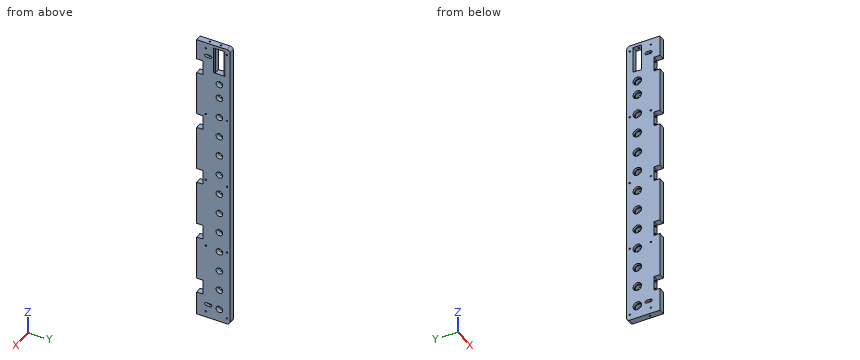
```python
from build123d import *

# Parameters (mm, degrees)
SKETCH1_W                 = 1000
SKETCH1_H                 = 100
SKETCH1_R                 = 11
SKETCH1_W_2               = 90
SKETCH1_H_2               = 28
BOSS_EXTRUDE1_DEPTH       = 20
SKETCH2_W                 = 20
SKETCH2_H                 = 50
SKETCH2_R                 = 4
CUT_EXTRUDE2_DEPTH        = 20
LPATTERN1_COUNT           = 2
LPATTERN1_PITCH           = 220
SKETCH12_R                = 14
CUT_EXTRUDE6_DEPTH        = 8
SKETCH14_W                = 2.5
SKETCH14_H                = 10
SKETCH16_W                = 90
SKETCH16_H                = 5
CUT_EXTRUDE7_DEPTH        = 3
SKETCH17_W                = 90
SKETCH17_H                = 5
CUT_EXTRUDE8_DEPTH        = 3
SKETCH18_R                = 14
CUT_EXTRUDE9_DEPTH        = 8
SKETCH20_W                = 20
SKETCH20_H                = 1000
BOSS_EXTRUDE2_DEPTH       = 10
FILLET1_R                 = 10
FILLET2_R                 = 10
F_5_0MM_DOWEL_HOLE3_D     = 5
F_5_0MM_DOWEL_HOLE3_DEPTH = 10
F_5_0MM_DOWEL_HOLE3_TIP   = 1.502151548
SKETCH27_R                = 2.5
CUT_EXTRUDE10_DEPTH       = 55
CUT_EXTRUDE11_DEPTH       = 1035.26302264
CUT_EXTRUDE12_START       = -70
SKETCH29_R                = 2.5
CUT_EXTRUDE12_DEPTH       = 70
SKETCH30_R                = 2.5
CUT_EXTRUDE13_DEPTH       = 1035.26302264
CUT_EXTRUDE14_REACH       = 1036.263
SKETCH31_W                = 1251.907534991
SKETCH31_H                = 393.114099754
SKETCH32_R                = 4
CUT_EXTRUDE15_DEPTH       = 35


with BuildPart() as part:
    # Sketch1 → Boss-Extrude1 (new body)
    with BuildSketch(Plane(origin=(0, 0, 0), x_dir=(0, 0, -1), z_dir=(1, 0, 0))):
        with Locations((500, 50)):
            Rectangle(SKETCH1_W, SKETCH1_H)
        with Locations((956.5, 75)):
            Circle(SKETCH1_R, mode=Mode.SUBTRACT)
        with Locations((886.5, 75)):
            Circle(SKETCH1_R, mode=Mode.SUBTRACT)
        with Locations((816.5, 75)):
            Circle(SKETCH1_R, mode=Mode.SUBTRACT)
        with Locations((746.5, 75)):
            Circle(SKETCH1_R, mode=Mode.SUBTRACT)
        with Locations((676.5, 75)):
            Circle(SKETCH1_R, mode=Mode.SUBTRACT)
        with Locations((606.5, 75)):
            Circle(SKETCH1_R, mode=Mode.SUBTRACT)
        with Locations((536.5, 75)):
            Circle(SKETCH1_R, mode=Mode.SUBTRACT)
        with Locations((466.5, 75)):
            Circle(SKETCH1_R, mode=Mode.SUBTRACT)
        with Locations((396.5, 75)):
            Circle(SKETCH1_R, mode=Mode.SUBTRACT)
        with Locations((326.5, 75)):
            Circle(SKETCH1_R, mode=Mode.SUBTRACT)
        with Locations((256.5, 75)):
            Circle(SKETCH1_R, mode=Mode.SUBTRACT)
        with Locations((186.5, 75)):
            Circle(SKETCH1_R, mode=Mode.SUBTRACT)
        with Locations((136.5, 75)):
            Circle(SKETCH1_R, mode=Mode.SUBTRACT)
        with Locations((55, 75)):
            Rectangle(SKETCH1_W_2, SKETCH1_H_2, mode=Mode.SUBTRACT)
    extrude(amount=BOSS_EXTRUDE1_DEPTH)

    # Sketch2 → Cut-Extrude2 (cut)
    # profile 1 of 5: a face of its own
    with BuildSketch(Plane.XZ):
        with Locations((10, -895)):
            Rectangle(SKETCH2_W, SKETCH2_H)
        with Locations(Location((10, -910, 0), (0, 0, 270))):
            Circle(SKETCH2_R, mode=Mode.SUBTRACT)
        with Locations(Location((10, -880, 0), (0, 0, 270))):
            Circle(SKETCH2_R, mode=Mode.SUBTRACT)
    # profile 2 of 5: a face of its own
    with BuildSketch(Plane.XZ):
        with Locations((10, -695)):
            Rectangle(SKETCH2_W, SKETCH2_H)
        with Locations(Location((10, -710, 0), (0, 0, 270))):
            Circle(SKETCH2_R, mode=Mode.SUBTRACT)
        with Locations(Location((10, -680, 0), (0, 0, 270))):
            Circle(SKETCH2_R, mode=Mode.SUBTRACT)
    # profile 3 of 5: a face of its own
    with BuildSketch(Plane.XZ):
        with Locations((10, -495)):
            Rectangle(SKETCH2_W, SKETCH2_H)
        with Locations(Location((10, -510, 0), (0, 0, 270))):
            Circle(SKETCH2_R, mode=Mode.SUBTRACT)
        with Locations(Location((10, -480, 0), (0, 0, 270))):
            Circle(SKETCH2_R, mode=Mode.SUBTRACT)
    # profile 4 of 5: a face of its own
    with BuildSketch(Plane.XZ):
        with Locations((10, -295)):
            Rectangle(SKETCH2_W, SKETCH2_H)
        with Locations(Location((10, -310, 0), (0, 0, 270))):
            Circle(SKETCH2_R, mode=Mode.SUBTRACT)
        with Locations(Location((10, -280, 0), (0, 0, 270))):
            Circle(SKETCH2_R, mode=Mode.SUBTRACT)
    # profile 5 of 5: a face of its own
    with BuildSketch(Plane.XZ):
        with Locations((10, -95)):
            Rectangle(SKETCH2_W, SKETCH2_H)
        with Locations(Location((10, -110, 0), (0, 0, 270))):
            Circle(SKETCH2_R, mode=Mode.SUBTRACT)
        with Locations(Location((10, -80, 0), (0, 0, 270))):
            Circle(SKETCH2_R, mode=Mode.SUBTRACT)
    extrude(amount=-CUT_EXTRUDE2_DEPTH, mode=Mode.SUBTRACT)


with BuildPart() as lpattern1_1:
    # LPattern1: pattern copy
    add(part.part.moved(Location(Vector(-1, 0, 0) * (1 * LPATTERN1_PITCH))))

    # Sketch12 → Cut-Extrude6 (cut)
    with BuildSketch(Plane(origin=(-200, 0, 0), x_dir=(0, 0, -1), z_dir=(1, 0, 0))):
        with Locations((956.5, 75)):
            Circle(SKETCH12_R)
        with Locations((886.5, 75)):
            Circle(SKETCH12_R)
        with Locations((816.5, 75)):
            Circle(SKETCH12_R)
        with Locations((746.5, 75)):
            Circle(SKETCH12_R)
        with Locations((676.5, 75)):
            Circle(SKETCH12_R)
        with Locations((606.5, 75)):
            Circle(SKETCH12_R)
        with Locations((536.5, 75)):
            Circle(SKETCH12_R)
        with Locations((466.5, 75)):
            Circle(SKETCH12_R)
        with Locations((396.5, 75)):
            Circle(SKETCH12_R)
        with Locations((326.5, 75)):
            Circle(SKETCH12_R)
        with Locations((256.5, 75)):
            Circle(SKETCH12_R)
        with Locations((186.5, 75)):
            Circle(SKETCH12_R)
        with Locations((136.5, 75)):
            Circle(SKETCH12_R)
    extrude(amount=-CUT_EXTRUDE6_DEPTH, mode=Mode.SUBTRACT)

    # Sketch16 → Cut-Extrude7 (cut)
    with BuildSketch(Plane.ZY.offset(220)):
        with Locations((-55, 91.5)):
            Rectangle(SKETCH16_W, SKETCH16_H)
        with Locations((-55, 58.5)):
            Rectangle(SKETCH16_W, SKETCH16_H)
    extrude(amount=-CUT_EXTRUDE7_DEPTH, mode=Mode.SUBTRACT)


with BuildPart() as part_1:
    add(part.part)

    # Sketch14 → Ø5.0mm Dowel Hole1 (revolve, cut)
    with BuildSketch(Plane(origin=(10, 75, 0), x_dir=(0, -1, 0), z_dir=(1, 0, 0))):
        with Locations((1.25, 5)):
            Rectangle(SKETCH14_W, SKETCH14_H)
    revolve(axis=Axis((10, 75, 6.35), (0, 0, -1)), mode=Mode.SUBTRACT)

    # Sketch17 → Cut-Extrude8 (cut)
    with BuildSketch(Plane(origin=(20, 0, 0), x_dir=(0, 0, -1), z_dir=(1, 0, 0))):
        with Locations((55, 91.5)):
            Rectangle(SKETCH17_W, SKETCH17_H)
        with Locations((55, 58.5)):
            Rectangle(SKETCH17_W, SKETCH17_H)
    extrude(amount=-CUT_EXTRUDE8_DEPTH, mode=Mode.SUBTRACT)

    # Sketch18 → Cut-Extrude9 (cut)
    with BuildSketch(Plane.ZY):
        with Locations((-956.5, 75)):
            Circle(SKETCH18_R)
        with Locations((-886.5, 75)):
            Circle(SKETCH18_R)
        with Locations((-816.5, 75)):
            Circle(SKETCH18_R)
        with Locations((-746.5, 75)):
            Circle(SKETCH18_R)
        with Locations((-676.5, 75)):
            Circle(SKETCH18_R)
        with Locations((-606.5, 75)):
            Circle(SKETCH18_R)
        with Locations((-536.5, 75)):
            Circle(SKETCH18_R)
        with Locations((-466.5, 75)):
            Circle(SKETCH18_R)
        with Locations((-396.5, 75)):
            Circle(SKETCH18_R)
        with Locations((-326.5, 75)):
            Circle(SKETCH18_R)
        with Locations((-256.5, 75)):
            Circle(SKETCH18_R)
        with Locations((-186.5, 75)):
            Circle(SKETCH18_R)
        with Locations((-136.5, 75)):
            Circle(SKETCH18_R)
    extrude(amount=-CUT_EXTRUDE9_DEPTH, mode=Mode.SUBTRACT)

    add(lpattern1_1.part)  # Boss-Extrude2 merges LPattern1_1
    # Sketch20 → Boss-Extrude2 (add)
    with BuildSketch(Plane(origin=(0, 100, 0), x_dir=(1, 0, 0), z_dir=(0, 1, 0))):
        with Locations((-210, 500)):
            Rectangle(SKETCH20_W, SKETCH20_H)
        with Locations((10, 500)):
            Rectangle(SKETCH20_W, SKETCH20_H)
    extrude(amount=BOSS_EXTRUDE2_DEPTH)

    # Fillet1
    fillet1_edges = [part_1.edges().sort_by_distance(p)[0] for p in [
        (-210, 110, 0),
        (-210, 110, -1000),
    ]]
    fillet(fillet1_edges, radius=FILLET1_R)

    # Fillet2
    fillet2_edges = [part_1.edges().sort_by_distance(p)[0] for p in [
        (10, 110, 0),
        (10, 110, -1000),
    ]]
    fillet(fillet2_edges, radius=FILLET2_R)

    # Ø5.0mm Dowel Hole3
    with Locations(Plane(origin=(-210, 74.987891575, 0), x_dir=(1, 0, 0), z_dir=(0, 0, 1))):
        with Locations((0, 0)):
            Hole(F_5_0MM_DOWEL_HOLE3_D / 2, depth=F_5_0MM_DOWEL_HOLE3_DEPTH)
            with Locations((0, 0, -(F_5_0MM_DOWEL_HOLE3_DEPTH + F_5_0MM_DOWEL_HOLE3_TIP / 2))):  # 118° drill point
                Cone(0, F_5_0MM_DOWEL_HOLE3_D / 2, F_5_0MM_DOWEL_HOLE3_TIP, mode=Mode.SUBTRACT)

    # Sketch27 → Cut-Extrude10 (cut)
    with BuildSketch(Plane.XY):
        with Locations((-210, 38)):
            Circle(SKETCH27_R)
        with Locations((10, 38)):
            Circle(SKETCH27_R)
    extrude(amount=-CUT_EXTRUDE10_DEPTH, mode=Mode.SUBTRACT)

    # Sketch28 → Cut-Extrude11 (cut, through all)
    with BuildSketch(Plane.ZY.offset(220)):
        with BuildLine():
            Line((-42, 44.831263619), (-42, 31.168736381))
            ThreePointArc((-42, 31.168736381), (-47, 26.168736381), (-52, 31.168736381))
            Line((-52, 31.168736381), (-52, 44.831263619))
            ThreePointArc((-52, 44.831263619), (-47, 49.831263619), (-42, 44.831263619))
        make_face()
        with BuildLine():
            Line((-958, 44.831263619), (-958, 31.168736381))
            ThreePointArc((-958, 31.168736381), (-953, 26.168736381), (-948, 31.168736381))
            Line((-948, 31.168736381), (-948, 44.831263619))
            ThreePointArc((-948, 44.831263619), (-953, 49.831263619), (-958, 44.831263619))
        make_face()
    extrude(amount=-CUT_EXTRUDE11_DEPTH, mode=Mode.SUBTRACT)

    # Sketch29 → Cut-Extrude12 (cut)
    with BuildSketch(Plane(origin=(0, 0, -1000), x_dir=(-1, 0, 0), z_dir=(0, 0, -1)).offset(CUT_EXTRUDE12_START)):
        with Locations(Location((-10, 38, 0), (0, 0, 180))):
            Circle(SKETCH29_R)
        with Locations(Location((210, 38, 0), (0, 0, 180))):
            Circle(SKETCH29_R)
    extrude(amount=CUT_EXTRUDE12_DEPTH, mode=Mode.SUBTRACT)

    # Sketch30 → Cut-Extrude13 (cut, through all)
    with BuildSketch(Plane(origin=(20, 0, 0), x_dir=(0, 0, -1), z_dir=(1, 0, 0))):
        with Locations((500, 30)):
            Circle(SKETCH30_R)
        with Locations((20, 30)):
            Circle(SKETCH30_R)
        with Locations((20, 100)):
            Circle(SKETCH30_R)
        with Locations((500, 100)):
            Circle(SKETCH30_R)
        with Locations((980, 100)):
            Circle(SKETCH30_R)
        with Locations((980, 30)):
            Circle(SKETCH30_R)
        with Locations((260, 100)):
            Circle(SKETCH30_R)
        with Locations((740, 100)):
            Circle(SKETCH30_R)
        with Locations((740, 30)):
            Circle(SKETCH30_R)
        with Locations((260, 30)):
            Circle(SKETCH30_R)
    extrude(amount=-CUT_EXTRUDE13_DEPTH, mode=Mode.SUBTRACT)

    # Sketch31 → Cut-Extrude14 (cut, up to next)
    with BuildSketch(Plane.ZY.offset(220), mode=Mode.PRIVATE) as cut_extrude14_sk1:
        with Locations((-530.819455446, 0)):
            Rectangle(SKETCH31_W, SKETCH31_H)
    cut_extrude14_tool1 = extrude(cut_extrude14_sk1.sketch, amount=-CUT_EXTRUDE14_REACH, mode=Mode.PRIVATE) & part_1.part
    add(cut_extrude14_tool1.solids().sort_by_distance((-220, 0, -530.819455))[0], mode=Mode.SUBTRACT)

    # Sketch32 → Cut-Extrude15 (cut)
    with BuildSketch(Plane.XZ):
        with Locations(Location((10, -310, 0), (0, 0, 270))):
            Circle(SKETCH32_R)
        with Locations(Location((10, -280, 0), (0, 0, 270))):
            Circle(SKETCH32_R)
        with Locations(Location((10, -110, 0), (0, 0, 270))):
            Circle(SKETCH32_R)
        with Locations(Location((10, -80, 0), (0, 0, 270))):
            Circle(SKETCH32_R)
        with Locations(Location((10, -480, 0), (0, 0, 270))):
            Circle(SKETCH32_R)
        with Locations(Location((10, -510, 0), (0, 0, 270))):
            Circle(SKETCH32_R)
        with Locations(Location((10, -680, 0), (0, 0, 270))):
            Circle(SKETCH32_R)
        with Locations(Location((10, -710, 0), (0, 0, 270))):
            Circle(SKETCH32_R)
        with Locations(Location((10, -880, 0), (0, 0, 270))):
            Circle(SKETCH32_R)
        with Locations(Location((10, -910, 0), (0, 0, 270))):
            Circle(SKETCH32_R)
    extrude(amount=-CUT_EXTRUDE15_DEPTH, mode=Mode.SUBTRACT)


solid = part_1.part
```
Work out the finished part from the listing and answer in its coordinate system (mm). Coordinates: 2 decimals unless noted, no trailing zeros. Order: outer loops, then holes, each group sorted by start corner. A loop starts at its lowest first (then second) coordinate and runs counter-clockwise, first axis right, second up. Notation, with made-up numbers: (-21, 2) - (22, 2) arc R22 cw to (22, 30) - close; hole circle Ø7 at (71, -2.5). An arc over 180 degrees is marked (long way). Answer as a JSON object with one key per item and string values.
1. Find section A-A on z = -136.5. Determine the outline of the cut face in (x, y).
Output values:
{"outline": "(0, 0) - (20, 0) - (20, 64) - (8, 64) - (8, 61) - (0, 61) - close; (0, 89) - (8, 89) - (8, 86) - (20, 86) - (20, 110) - (0, 110) - close"}
2. Each of these flat-tipped pins is pushed along its axis until it touches: P1, Ø1.5, axis at x = 10.5, y = 38.5, coming from the -Z side; P2, Ø10.5, axis at x = 10, z = -680, coming from the -Y side; P3, Ø4.5, axis at y = 100, z = -260, coming from the +X side; P4, Ø14, axis at y = 76, z = -963, coming from the -X side. Where does it stop, or does it pass through?
Output values:
{"P1": "stops at z = -930", "P2": "stops at y = 20", "P3": "passes through", "P4": "stops at x = 8"}
3. Consider line 1 (Z direction, x = 1.25, y = 8.5); line 2 (Y direction, x = 3.5, z = -95.5); line 3 (Z direction, x = 16.75, y = 40.5). Determine where each line is inside the solid, lowest interval first.
Output values:
{"line 1": "z = -1000 to -920, -870 to -720, -670 to -520, -470 to -320, -270 to -120, -70 to 0", "line 2": "y = 20 to 61, 89 to 110", "line 3": "z = -1000 to -958, -948 to -52, -42 to 0"}
